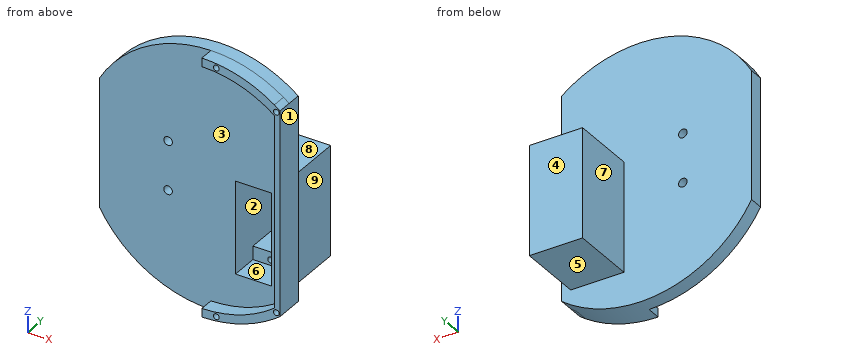
from build123d import *

# Parameters (mm, degrees)
SKETCH_1_R          = 1.5
EXTRUDE_1_DEPTH     = 5
SKETCH_3_W          = 18.6
SKETCH_3_H          = 38.3
SKETCH_3_W_2        = 12.6
SKETCH_3_H_2        = 32.3
EXTRUDE_3_DEPTH     = 19.8
SKETCH_4_W          = 18.6
SKETCH_4_H          = 38.3
EXTRUDE_4_DEPTH     = 3
SKETCH_7_W          = 12.6
SKETCH_7_H          = 32.3
CUT_EXTRUDE_1_DEPTH = 5
SKETCH_8_W          = 35.927581395
SKETCH_8_H          = 53.234071865
CUT_EXTRUDE_2_DEPTH = 14.8
SKETCH_9_W          = 12.6
SKETCH_9_H          = 4.7
EXTRUDE_5_DEPTH     = 15.2
SKETCH_10_R         = 1.1
CUT_EXTRUDE_3_DEPTH = 10
EXTRUDE_6_DEPTH     = 5
SKETCH_13_R         = 1
CUT_EXTRUDE_4_DEPTH = 5


with BuildPart() as part:
    # 草图1 → 凸台-拉伸1 (new body)
    with BuildSketch(Plane(origin=(0, 0, 0), x_dir=(1, 0, 0), z_dir=(0, 1, 0))):
        with BuildLine():
            Line((-39.038561358, -22.382822144), (-39.038561358, 22.382822144))
            ThreePointArc((-39.038561358, 22.382822144), (-8.857541047, 44.119655105), (27.374530931, 35.716033603))
            Line((27.374530931, 35.716033603), (27.374530931, -35.716033603))
            ThreePointArc((27.374530931, -35.716033603), (-8.857541047, -44.119655105), (-39.038561358, -22.382822144))
        make_face()
        with Locations((-15, 8.55)):
            Circle(SKETCH_1_R, mode=Mode.SUBTRACT)
        with Locations((-15, -8.55)):
            Circle(SKETCH_1_R, mode=Mode.SUBTRACT)
    extrude(amount=EXTRUDE_1_DEPTH)

    # 草图3 → 凸台-拉伸3 (add, symmetric)
    with BuildSketch(Plane(origin=(0, 5, 0), x_dir=(1, 0, 0), z_dir=(0, 1, 0))):
        with Locations((14.904530931, 13.65)):
            Rectangle(SKETCH_3_W, SKETCH_3_H)
        with Locations((14.904530931, 13.65)):
            Rectangle(SKETCH_3_W_2, SKETCH_3_H_2, mode=Mode.SUBTRACT)
    extrude(amount=EXTRUDE_3_DEPTH, both=True)

    # 草图4 → 凸台-拉伸4 (add)
    with BuildSketch(Plane(origin=(0, 24.8, 0), x_dir=(1, 0, 0), z_dir=(0, 1, 0))):
        with Locations((14.904530931, 13.65)):
            Rectangle(SKETCH_4_W, SKETCH_4_H)
    extrude(amount=EXTRUDE_4_DEPTH)

    # 草图7 → 切除-拉伸1 (cut)
    with BuildSketch(Plane(origin=(0, 0, 0), x_dir=(-1, 0, 0), z_dir=(0, -1, 0))):
        with Locations((-14.904530931, 13.65)):
            Rectangle(SKETCH_7_W, SKETCH_7_H)
    extrude(amount=-CUT_EXTRUDE_1_DEPTH, mode=Mode.SUBTRACT)

    # 草图8 → 切除-拉伸2 (cut)
    with BuildSketch(Plane(origin=(0, -14.8, 0), x_dir=(-1, 0, 0), z_dir=(0, -1, 0))):
        with Locations((-13.744141361, 17.136677553)):
            Rectangle(SKETCH_8_W, SKETCH_8_H)
    extrude(amount=-CUT_EXTRUDE_2_DEPTH, mode=Mode.SUBTRACT)

    # 草图9 → 凸台-拉伸5 (add)
    with BuildSketch(Plane.XZ.offset(-24.8)):
        with Locations((14.904530931, -27.45)):
            Rectangle(SKETCH_9_W, SKETCH_9_H)
    extrude_5 = extrude(amount=EXTRUDE_5_DEPTH)

    # 草图10 → 切除-拉伸3 (cut)
    with BuildSketch(Plane(origin=(0, 9.6, 0), x_dir=(-1, 0, 0), z_dir=(0, -1, 0))):
        with Locations((-14.904530931, 27.9)):
            Circle(SKETCH_10_R)
    cut_extrude_3 = extrude(amount=-CUT_EXTRUDE_3_DEPTH, mode=Mode.SUBTRACT)

    # 镜向1: 凸台-拉伸5, 切除-拉伸3 across plane
    add(extrude_5.mirror(Plane.XY.offset(-13.65)))
    add(cut_extrude_3.mirror(Plane.XY.offset(-13.65)), mode=Mode.SUBTRACT)

    # 草图11 → 凸台-拉伸6 (add)
    with BuildSketch(Plane(origin=(0, 0, 0), x_dir=(-1, 0, 0), z_dir=(0, -1, 0))):
        with BuildLine():
            Line((0, 42), (0, 45))
            ThreePointArc((0, 45), (-13.278516311, 42.996290591), (-25.374530931, 37.163600203))
            Line((-25.374530931, 37.163600203), (-25.374530931, 33.46839076))
            ThreePointArc((-25.374530931, 33.46839076), (-13.385208031, 39.810001331), (0, 42))
        make_face()
        with BuildLine():
            Line((0, -45), (0, -42))
            ThreePointArc((0, -42), (-13.385208031, -39.810001331), (-25.374530931, -33.46839076))
            Line((-25.374530931, -33.46839076), (-25.374530931, -37.163600203))
            ThreePointArc((-25.374530931, -37.163600203), (-13.278516311, -42.996290591), (0, -45))
        make_face()
        with BuildLine():
            Line((-25.374530931, 33.46839076), (-25.374530931, 37.163600203))
            ThreePointArc((-25.374530931, 37.163600203), (-26.384460277, 36.453535575), (-27.374530931, 35.716033603))
            Line((-27.374530931, 35.716033603), (-27.374530931, 31.853336659))
            ThreePointArc((-27.374530931, 31.853336659), (-26.386890339, 32.676168965), (-25.374530931, 33.46839076))
        make_face()
        with BuildLine():
            Line((-25.374530931, -37.163600203), (-25.374530931, -33.46839076))
            ThreePointArc((-25.374530931, -33.46839076), (-26.386890339, -32.676168965), (-27.374530931, -31.853336659))
            Line((-27.374530931, -31.853336659), (-27.374530931, -35.716033603))
            ThreePointArc((-27.374530931, -35.716033603), (-26.384460277, -36.453535575), (-25.374530931, -37.163600203))
        make_face()
        with BuildLine():
            Line((-25.374530931, -33.46839076), (-25.374530931, 33.46839076))
            ThreePointArc((-25.374530931, 33.46839076), (-26.386890339, 32.676168965), (-27.374530931, 31.853336659))
            Line((-27.374530931, 31.853336659), (-27.374530931, -31.853336659))
            ThreePointArc((-27.374530931, -31.853336659), (-26.386890339, -32.676168965), (-25.374530931, -33.46839076))
        make_face()
        with BuildLine():
            Line((-25.374530931, 33.46839076), (-25.374530931, 37.163600203))
            ThreePointArc((-25.374530931, 37.163600203), (-26.384460277, 36.453535575), (-27.374530931, 35.716033603))
            Line((-27.374530931, 35.716033603), (-27.374530931, 31.853336659))
            ThreePointArc((-27.374530931, 31.853336659), (-26.386890339, 32.676168965), (-25.374530931, 33.46839076))
        make_face()
        with BuildLine():
            Line((-25.374530931, -37.163600203), (-25.374530931, -33.46839076))
            ThreePointArc((-25.374530931, -33.46839076), (-26.386890339, -32.676168965), (-27.374530931, -31.853336659))
            Line((-27.374530931, -31.853336659), (-27.374530931, -35.716033603))
            ThreePointArc((-27.374530931, -35.716033603), (-26.384460277, -36.453535575), (-25.374530931, -37.163600203))
        make_face()
        with BuildLine():
            Line((0, 42), (0, 45))
            ThreePointArc((0, 45), (-13.278516311, 42.996290591), (-25.374530931, 37.163600203))
            Line((-25.374530931, 37.163600203), (-25.374530931, 33.46839076))
            ThreePointArc((-25.374530931, 33.46839076), (-13.385208031, 39.810001331), (0, 42))
        make_face()
        with BuildLine():
            Line((0, -45), (0, -42))
            ThreePointArc((0, -42), (-13.385208031, -39.810001331), (-25.374530931, -33.46839076))
            Line((-25.374530931, -33.46839076), (-25.374530931, -37.163600203))
            ThreePointArc((-25.374530931, -37.163600203), (-13.278516311, -42.996290591), (0, -45))
        make_face()
    extrude(amount=EXTRUDE_6_DEPTH)

    # 草图13 → 切除-拉伸4 (cut)
    with BuildSketch(Plane(origin=(0, -5, 0), x_dir=(-1, 0, 0), z_dir=(0, -1, 0))):
        with Locations((-5.074530931, 43.202999153)):
            Circle(SKETCH_13_R)
        with Locations((-26.074530931, 34.819087247)):
            Circle(SKETCH_13_R)
        with Locations((-26.074530931, -34.819087247)):
            Circle(SKETCH_13_R)
        with Locations((-5.074530931, -43.202999153)):
            Circle(SKETCH_13_R)
    extrude(amount=-CUT_EXTRUDE_4_DEPTH, mode=Mode.SUBTRACT)


solid = part.part
CAD build for the part. Positions are in the model's coordinates, mm. Face numbers are marked on the shaded views. A direction names the side the tool comes from. Give positions to 0.01 mm unless a question says otherwise; leave off trailing zeros. Loops run counter-clockwise (first coordinate to the right, second up) from the corner with the lowest first, then second, coordinate; pieces in that order, holes last. Notation, with made-up numbers: M -10.5,82 L 41.5,82 A19 cw 41.5,104 Z; hole C 21,-5.75 d5. An arc over 180 degrees is marked long. Answer in a Markdown table with one row per item. Add a question column.
Item 1: Band-saw the part on A-A on y = 16. Give the cut face in (x, z).
Item 2: Mould opens along X. For the marked faces 6, 7, 8 and 9 say: +X half, -X half, draft (parallel to the pull), parting line (faces both ways), or undercut.
Item 3: Band-saw the part on C-C on z = 8.55. Give the cut face in (x, y), then the cut area to 3 significant figures.
Item 4: Drop flat-ended pins along their axis: P1, Ø9.5, axis at x = 16.5, y = 18, coming from the -Z side; P2, Ø2.5, axis at x = 26.07, z = 34.82, coming from the +Y side; P3, Ø1.5, axis at y = -3.5, z = -43, coming from the -X side; P4, Ø12.5, axis at y = 11, z = -18.5, coming from the +X side. Give the stop position or say it passes through.
Item 5: Band-saw the part on B-B on z = -3.5. Give the cut face in (x, y).
Item 6: Band-saw the part on D-D on y = 8. Give the cut face in (x, z), then the cut area to 3 significant figures.
Item 7: Probe probe 1 along X at (y, z) = (20, -13); probe 2 along Z at (x, y) = (15, 14); probe 3 along Z at (x, y) = (-15, 1.8). List the from-to ranges inside material, lowest first.
Item 8: Tool access for the marked faces 1, 2, 3, 4 and 5: list every direction of +Z, -Z, +X, -X, +Y, -Y with a clear straight run to the whole face (end or side of a thin tool).
Reply:
| question | item | result |
|---|---|---|
| 1 | outline | M 5.6,-32.8 L 24.2,-32.8 L 24.2,5.5 L 5.6,5.5 Z; hole M 8.6,-25.1 L 21.2,-25.1 L 21.2,-2.2 L 8.6,-2.2 Z; hole C 14.9,-27.9 d2.2; hole C 14.9,0.6 d2.2 |
| 2 | face 6 | undercut |
| 2 | face 7 | -X half |
| 2 | face 8 | draft |
| 2 | face 9 | +X half |
| 3 | outline | M -39.04,0 L -16.5,0 L -16.5,5 L -39.04,5 Z; M -13.5,0 L 25.37,0 L 25.37,-5 L 27.37,-5 L 27.37,5 L -13.5,5 Z |
| 3 | area | 327 mm^2 |
| 4 | P1 | stops at z = -32.8 |
| 4 | P2 | stops at y = 5 |
| 4 | P3 | stops at x = 0 |
| 4 | P4 | stops at x = 27.37 |
| 5 | outline | M -39.04,0 L 8.6,0 L 8.6,24.8 L 21.2,24.8 L 21.2,0 L 25.37,0 L 25.37,-5 L 27.37,-5 L 27.37,5 L 24.2,5 L 24.2,27.8 L 5.6,27.8 L 5.6,5 L -39.04,5 Z |
| 6 | outline | M 5.6,-32.8 L 24.2,-32.8 L 24.2,5.5 L 5.6,5.5 Z; hole M 8.6,-29.8 L 21.2,-29.8 L 21.2,2.5 L 8.6,2.5 Z |
| 6 | area | 305 mm^2 |
| 7 | probe 1 | x = 5.6 to 8.6, 21.2 to 24.2 |
| 7 | probe 2 | z = -32.8 to -29, -26.8 to -25.1, -2.2 to -0.5, 1.7 to 5.5 |
| 7 | probe 3 | z = -42.43 to -10.05, -7.05 to 7.05, 10.05 to 42.43 |
| 8 | face 1 | +Z, -Z, +X, +Y, -Y |
| 8 | face 2 | -Y |
| 8 | face 3 | -X, -Y |
| 8 | face 4 | +Z, -Z, +X, -X, +Y |
| 8 | face 5 | -Z, +X, -X, +Y |
